Geometry: final body of the model. Coordinates: model frame, mm. Face numbers are marked on the shaded views. Give positions to 0.01 mm unless a question says otherwise; leave off trailing zeros. Write each loop counter-clockwise with the first axis right and the second up, starting at its lowest first coordinate (ties: lowest second). Pieces come first, ordered by that corner, then holes. Notation, with made-up numbers: (48, 42.25) -> (85, 42.25) arc R11 ccw to (85, 52.25) -> close; hole circle Ø7 at (68.25, 24). An arc over 180 degrees is marked (long way). Answer as a JSON object with one key per item and string values.
from build123d import *

# Parameters (mm, degrees)
SKETCH1_R           = 3
SKETCH1_R_2         = 2
BOSS_EXTRUDE1_DEPTH = 4
SKETCH2_R           = 6
BOSS_EXTRUDE2_DEPTH = 4
SKETCH3_R           = 2
CUT_EXTRUDE1_DEPTH  = 9
CHAMFER1_SIZE       = 0.5


with BuildPart() as part:
    # Sketch1 → Boss-Extrude1 (new body)
    with BuildSketch(Plane.XY):
        with BuildLine():
            Line((-7.483314774, 13), (7.483314774, 13))
            ThreePointArc((7.483314774, 13), (0, -15), (-7.483314774, 13))
        make_face()
        with Locations((0, 8)):
            Circle(SKETCH1_R, mode=Mode.SUBTRACT)
        with Locations((-9, 0)):
            Circle(SKETCH1_R_2, mode=Mode.SUBTRACT)
        with Locations((11.144937976, 0)):
            Circle(SKETCH1_R_2, mode=Mode.SUBTRACT)
    extrude(amount=BOSS_EXTRUDE1_DEPTH)

    # Sketch2 → Boss-Extrude2 (add)
    with BuildSketch(Plane(origin=(0, 0, 0), x_dir=(-1, 0, 0), z_dir=(0, 0, -1))):
        with Locations((0, -5)):
            Circle(SKETCH2_R)
    extrude(amount=BOSS_EXTRUDE2_DEPTH)

    # Sketch3 → Cut-Extrude1 (cut, through all)
    with BuildSketch(Plane(origin=(0, 0, -4), x_dir=(-1, 0, 0), z_dir=(0, 0, -1))):
        with Locations((0, -5)):
            Circle(SKETCH3_R)
    extrude(amount=-CUT_EXTRUDE1_DEPTH, mode=Mode.SUBTRACT)

    # Chamfer1
    chamfer1_edges = [part.edges().sort_by_distance(p)[0] for p in [
        (6, -5, -4),
    ]]
    chamfer(chamfer1_edges, length=CHAMFER1_SIZE)


solid = part.part
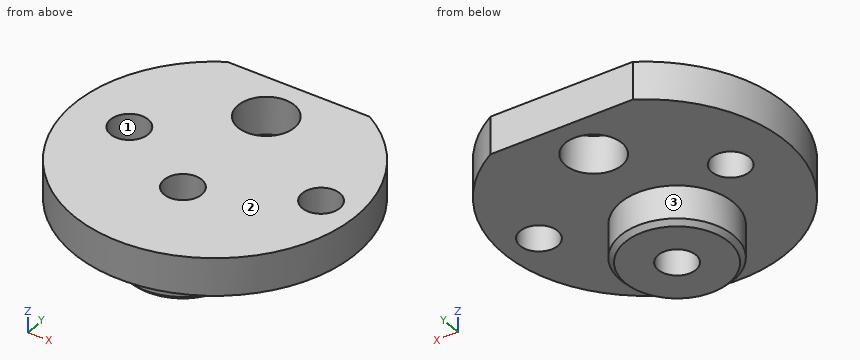
Q1. Material intervals for L1, parallel to Y at x = 0, z = -0.75; L2, parallel to Z at x = -3, y = 4.75; L3, parallel to Y at x = -9, z = 1.05, sorted ascending. Write a range as from..to.
Values:
{"L1": "-11..-7, -3..1", "L2": "0..4", "L3": "-12..-2, 2..12"}
Q2. Mould query, pull axis X, two halves, no side actions, for the marked faces 1, 2 and 3. Classes: pulls with the +X half, pulls with the -X half, needs draft (parallel to the pull), parting line crosses it, or undercut.
Values:
{"face 1": "undercut", "face 2": "needs draft", "face 3": "parting line crosses it"}
Q3. Cut plane B-B (y = 5.5). Return the cut outline in (x, z).
Values:
{"outline": "(-13.96, 0) -> (-1.66, 0) -> (-1.66, 4) -> (-13.96, 4) -> close; (1.66, 0) -> (13.96, 0) -> (13.96, 4) -> (1.66, 4) -> close"}
Q4. Cut plane A-A (x = 0). Return the cut outline in (y, z), and give its area (3 significant figures).
Values:
{"outline": "(-15, 0) -> (-11, 0) -> (-11, -3.5) -> (-10.5, -4) -> (-7, -4) -> (-7, 4) -> (-15, 4) -> close; (-3, -4) -> (0.5, -4) -> (1, -3.5) -> (1, 0) -> (5, 0) -> (5, 4) -> (-3, 4) -> close; (11, 0) -> (13, 0) -> (13, 4) -> (11, 4) -> close", "area": "104 mm²"}
Q5. Cut plane D-D (z = 1). Return the cut outline in (x, y), and give its area (3 significant figures).
Values:
{"outline": "(-7.48, 13) arc R15 ccw (long way) to (7.48, 13) -> close; hole circle Ø4 at (-9, 0); hole circle Ø6 at (0, 8); hole circle Ø4 at (0, -5); hole circle Ø4 at (11.14, 0)", "area": "621 mm²"}
Q6. Cut plane C-C (z = -2.25). Return the cut outline in (x, y), and give its area (3 significant figures).
Values:
{"outline": "circle Ø12 at (0, -5); hole circle Ø4 at (0, -5)", "area": "101 mm²"}
Q7. First-contact query: P1, Ø3, axis at x = -11.5, z = -3, coming from the -Y side; P2, Ø4.5, axis at x = 11.14, y = 0, coming from the -Z side; P3, Ø1.5, axis at y = -6, z = -1, coming from the -X side; P4, Ø2, axis at x = 3, z = 0, coming from the -Y side. Flat tips, straight axial feed; report the tip coordinate or a pass-through.
Values:
{"P1": "through", "P2": "z = 0", "P3": "x = -5.99", "P4": "y = -14.87"}
